CAD build for the part. Positions are in the model's coordinates, mm. A direction names the side the tool comes from. Give positions to 0.01 mm unless a question says otherwise; leave off trailing zeros. Loops run counter-clockwise (first coordinate to the right, second up) from the corner with the lowest first, then second, coordinate; pieces in that order, holes last. Notation, with made-up numbers: M -39,45 L -27,45 A18 ccw -27,69 Z; hole C 7,38 d1. An arc over 180 degrees is marked long. One line per question, with ' | ' between items.
```python
from build123d import *

# Parameters (mm, degrees)
SKETCH1_W           = 63.7
SKETCH1_H           = 43.4
BOSS_EXTRUDE1_DEPTH = 1.6
SKETCH2_W           = 63.7
SKETCH2_H           = 43.4
SKETCH2_W_2         = 60.5
SKETCH2_H_2         = 40.2
BOSS_EXTRUDE2_DEPTH = 8
SKETCH4_W           = 60.5
SKETCH4_H           = 3
CUT_EXTRUDE1_DEPTH  = 54.421180257
SKETCH5_W           = 2.6
SKETCH5_H           = 5.5
CUT_EXTRUDE2_DEPTH  = 5
CHAMFER1_SIZE       = 2
FILLET1_R           = 1.6
CHAMFER2_SIZE       = 1.2


with BuildPart() as part:
    # Sketch1 → Boss-Extrude1 (new body)
    with BuildSketch(Plane.XY):
        Rectangle(SKETCH1_W, SKETCH1_H)
    extrude(amount=BOSS_EXTRUDE1_DEPTH)

    # Sketch2 → Boss-Extrude2 (add)
    with BuildSketch(Plane.XY.offset(1.6)):
        Rectangle(SKETCH2_W, SKETCH2_H)
        Rectangle(SKETCH2_W_2, SKETCH2_H_2, mode=Mode.SUBTRACT)
    extrude(amount=BOSS_EXTRUDE2_DEPTH)

    # Sketch4 → Cut-Extrude1 (cut, through all)
    with BuildSketch(Plane(origin=(0, -20.1, 0), x_dir=(1, 0, 0), z_dir=(0, 1, 0))):
        with Locations((0, -8.1)):
            Rectangle(SKETCH4_W, SKETCH4_H)
    extrude(amount=-CUT_EXTRUDE1_DEPTH, mode=Mode.SUBTRACT)

    # Sketch5 → Cut-Extrude2 (cut)
    with BuildSketch(Plane(origin=(0, 0, 0), x_dir=(-1, 0, 0), z_dir=(0, 0, -1))):
        with Locations((-30.55, -8.85)):
            Rectangle(SKETCH5_W, SKETCH5_H)
        with Locations((30.55, -8.85)):
            Rectangle(SKETCH5_W, SKETCH5_H)
    extrude(amount=-CUT_EXTRUDE2_DEPTH, mode=Mode.SUBTRACT)

    # Chamfer1
    # the kernel refuses this chamfer: 2 mm, written as the material it takes off along each edge
    with BuildSketch(Plane(origin=(-29.25, -6.1, 0), x_dir=(0.9996219169112968, 0, -0.02749587661058639), z_dir=(0, -1, 0))) as chamfer1_piece_1:
        Polygon((CHAMFER1_SIZE * 0.999621916911, CHAMFER1_SIZE * 0.0274958766106), (-CHAMFER1_SIZE * 0.0274958766106, CHAMFER1_SIZE * 0.999621916911), (0, 0), align=None)
    extrude(amount=5.5, mode=Mode.SUBTRACT)
    with BuildSketch(Plane(origin=(29.25, -6.1, 0), x_dir=(-0.9996219169112968, 0, -0.02749587661058639), z_dir=(0, -1, 0))) as chamfer1_piece_2:
        Polygon((CHAMFER1_SIZE * 0.999621916911, -CHAMFER1_SIZE * 0.0274958766106), (-CHAMFER1_SIZE * 0.0274958766106, -CHAMFER1_SIZE * 0.999621916911), (0, 0), align=None)
    extrude(amount=5.5, mode=Mode.SUBTRACT)

    # Fillet1
    fillet1_edges = [part.edges().sort_by_distance(p)[0] for p in [
        (-31.85, 21.7, 4.8),
        (-31.85, -21.7, 4.8),
        (31.85, -21.7, 4.8),
        (31.85, 21.7, 4.8),
    ]]
    fillet(fillet1_edges, radius=FILLET1_R)

    # Chamfer2
    chamfer2_edges = [part.edges().sort_by_distance(p)[0] for p in [
        (-31.85, 7, 0),
        (0, 21.7, 0),
        (31.85, -15.85, 0),
        (0, -21.7, 0),
        (31.38137085, 21.23137085, 0),
        (31.38137085, -21.23137085, 0),
        (-31.38137085, -21.23137085, 0),
        (-31.38137085, 21.23137085, 0),
        (-31.85, -15.85, 0),
        (31.85, 7, 0),
    ]]
    chamfer(chamfer2_edges, length=CHAMFER2_SIZE)


solid = part.part
```
Item 1: Mould opens along Y. For faces 1 (the flat face through (-31.24, 6.82, 0.59)), 2 (the flat face through (0, 20.1, 6)), 3 (the cylindrical face through (31.39, -21.22, 5.46)) say: pulls with the +Y half, pulls with the -Y half, needs draft (parallel to the pull), parting line crosses it, or undercut.
Conclusion:
face 1: needs draft | face 2: undercut | face 3: pulls with the -Y half
Item 2: Drop flat-ended pins along their axis: P1, Ø1.8, axis at x = 3, y = -21, coming from the +Z side; P2, Ø1, axis at x = -16.5, y = -15.5, coming from the +Z side; P3, Ø0.8, axis at x = 31, y = -10, coming from the -Z side. Give the stop position or say it passes through.
Conclusion:
P1: z = 6.6 | P2: z = 1.6 | P3: z = 5
Item 3: Saw through at D-D on y = 7. Give the cut face in (x, z).
Conclusion:
outline: M -31.85,1.2 L -30.65,0 L 30.65,0 L 31.85,1.2 L 31.85,9.6 L 30.25,9.6 L 30.25,1.6 L -30.25,1.6 L -30.25,9.6 L -31.85,9.6 Z
Item 4: Saw through at C-C on x = -7.5. Give the cut face in (y, z), and give its area (3 significant figures).
Conclusion:
outline: M -21.7,1.2 L -20.5,0 L 20.5,0 L 21.7,1.2 L 21.7,9.6 L 20.1,9.6 L 20.1,1.6 L -20.1,1.6 L -20.1,6.6 L -21.7,6.6 Z | area: 88.8 mm²
Item 5: 3-axis set-ups, long thin cutter, end or side, ignore diameter. For faces 4 (the flat face through (0, -20.1, 4)), 5 (the flat face through (-31, -6.1, 2)), 6 (the flat face through (0, 21, 9.6)), 7 (the flat face through (31, -9, 5)): which of +Z, -Z, +X, -X, +Y, -Y reach the whole face in a straight line?
Conclusion:
face 4: +Z | face 5: -Z, -X | face 6: +Z, +X, -X, +Y, -Y | face 7: -Z, +X, -X
Item 6: Saw through at B-B on z = 5.75. Give the cut face in (x, y), and give its area (3 significant figures).
Conclusion:
outline: M -31.85,-20.1 A1.6 ccw -30.25,-21.7 L 30.25,-21.7 A1.6 ccw 31.85,-20.1 L 31.85,20.1 A1.6 ccw 30.25,21.7 L -30.25,21.7 A1.6 ccw -31.85,20.1 Z; hole M -30.25,-20.1 L 30.25,-20.1 L 30.25,20.1 L -30.25,20.1 Z | area: 330 mm²
Item 7: Saw through at A-A on y = -9. Give the cut face in (x, z), and give its area (3 significant figures).
Conclusion:
outline: M -31.85,5 L -30.25,5 L -30.25,9.6 L -31.85,9.6 Z; M -28.85,1.6 L -27.25,0 L 27.25,0 L 28.85,1.6 Z; M 30.25,5 L 31.85,5 L 31.85,9.6 L 30.25,9.6 Z | area: 104 mm²
Item 8: Drill centre lines: line 1 along X through (y, z) = (2, 9.25); line 2 along Y through (x, z) = (-22, 2). Where is each one in solid material? Low to high. Write a range as [from, to].
Conclusion:
line 1: [-31.85, -30.25], [30.25, 31.85] | line 2: [-21.7, -20.1], [20.1, 21.7]
